Could you check a few things on this model? Use its own coordinates, in mm. Face numbers are marked on the shaded views. A direction names the side the tool comes from. Give positions to 0.01 mm unless a question says otherwise; leave off trailing zeros. Write each loop counter-clockwise with the first axis right and the second up, starting at its lowest first coordinate (ties: lowest second). Pieces come first, ordered by that corner, then holes. Notation, with made-up numbers: (37.25, 12) -> (63.25, 12) arc R22 ccw to (63.25, 28) -> close; hole circle Ø4 at (87.25, -10). An arc over 180 degrees is marked (long way). One line per question, with ' | ' between items.
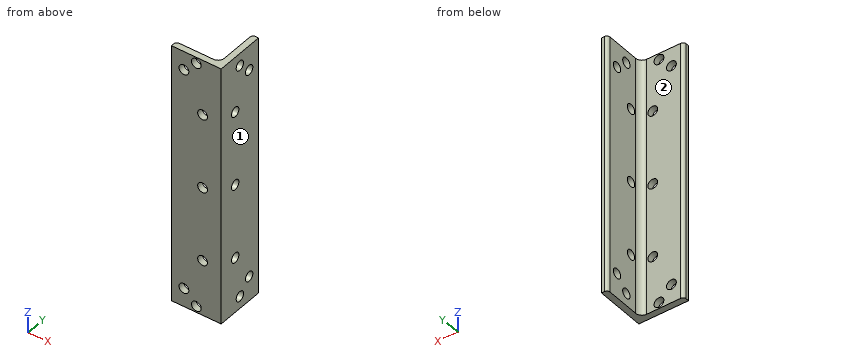
from build123d import *

# Parameters (mm, degrees)
BOSS_EXTRUDE1_DEPTH = 304.8
SKETCH7_W           = 25.4
SKETCH7_H           = 476.25
CUT_EXTRUDE1_DEPTH  = 254
SKETCH3_R           = 2.5
CUT_EXTRUDE2_DEPTH  = 254
SKETCH8_R           = 2.5
CUT_EXTRUDE4_DEPTH  = 254


with BuildPart() as part:
    # Sketch2 → Boss-Extrude1 (new, symmetric)
    with BuildSketch(Plane.XY):
        with BuildLine():
            Line((-12.7, -12.7), (12.7, -12.7))
            Line((12.7, -12.7), (12.7, 12.7))
            Line((12.7, 12.7), (11.1125, 12.7))
            ThreePointArc((11.1125, 12.7), (9.989967985, 12.235032015), (9.525, 11.1125))
            Line((9.525, 11.1125), (9.525, -6.35))
            ThreePointArc((9.525, -6.35), (8.59506403, -8.59506403), (6.35, -9.525))
            Line((6.35, -9.525), (-11.1125, -9.525))
            ThreePointArc((-11.1125, -9.525), (-12.235032015, -9.989967985), (-12.7, -11.1125))
            Line((-12.7, -11.1125), (-12.7, -12.7))
        make_face()
    extrude(amount=BOSS_EXTRUDE1_DEPTH, both=True)

    # Sketch7 → Cut-Extrude1 (cut)
    with BuildSketch(Plane.XZ.offset(12.7)):
        with Locations((0, 66.675)):
            Rectangle(SKETCH7_W, SKETCH7_H)
    extrude(amount=-CUT_EXTRUDE1_DEPTH, mode=Mode.SUBTRACT)

    # Sketch3 → Cut-Extrude2 (cut)
    with BuildSketch(Plane(origin=(0, 0, 0), x_dir=(1, 0, 0), z_dir=(0, 1, 0))):
        with Locations(Location((-6.35, 295.275, 0), (0, 0, 270))):
            Circle(SKETCH3_R)
        with Locations(Location((0, 301.625, 0), (0, 0, 270))):
            Circle(SKETCH3_R)
        with Locations(Location((3.175, 276.225, 0), (0, 0, 270))):
            Circle(SKETCH3_R)
        with Locations(Location((3.175, 238.125, 0), (0, 0, 270))):
            Circle(SKETCH3_R)
        with Locations(Location((3.175, 200.025, 0), (0, 0, 270))):
            Circle(SKETCH3_R)
        with Locations(Location((0, 174.625, 0), (0, 0, 270))):
            Circle(SKETCH3_R)
        with Locations(Location((-6.35, 180.975, 0), (0, 0, 270))):
            Circle(SKETCH3_R)
    extrude(amount=-CUT_EXTRUDE2_DEPTH, mode=Mode.SUBTRACT)

    # Sketch8 → Cut-Extrude4 (cut)
    with BuildSketch(Plane(origin=(12.7, 0, -12.7), x_dir=(0, 0, 1), z_dir=(-1, 0, 0))):
        with Locations(Location((-171.45, 6.35, 0), (0, 0, 90))):
            Circle(SKETCH8_R)
        with Locations(Location((-165.1, 0, 0), (0, 0, 90))):
            Circle(SKETCH8_R)
        with Locations(Location((-187.325, -3.175, 0), (0, 0, 90))):
            Circle(SKETCH8_R)
        with Locations(Location((-225.425, -3.175, 0), (0, 0, 90))):
            Circle(SKETCH8_R)
        with Locations(Location((-263.525, -3.175, 0), (0, 0, 90))):
            Circle(SKETCH8_R)
        with Locations(Location((-285.75, 0, 0), (0, 0, 90))):
            Circle(SKETCH8_R)
        with Locations(Location((-279.4, 6.35, 0), (0, 0, 90))):
            Circle(SKETCH8_R)
    extrude(amount=CUT_EXTRUDE4_DEPTH, mode=Mode.SUBTRACT)


solid = part.part
Q1. If I drill on line 1 along Y through (x, z) = (-8.5, -185) (3 decimals); line 2 along X through (y, z) = (4.25, -285) (3 decimals); line 3 along X through (y, z) = (-9.25, -277), over which ranges is the centre line in solid material (lowest first)?
Answer below:
line 1: y = -12.7 to -9.525 | line 2: x = 9.525 to 12.7 | line 3: x = 7.64 to 12.7
Q2. Imagine slicing it at B-B on x = -6.35. Please give me the cut outline in (y, z) (3 decimals), and give its area (3 significant figures).
Answer below:
outline: (-12.7, -304.8) -> (-9.525, -304.8) -> (-9.525, -297.775) -> (-12.7, -297.775) -> close; (-12.7, -292.775) -> (-9.525, -292.775) -> (-9.525, -183.475) -> (-12.7, -183.475) -> close; (-12.7, -178.475) -> (-9.525, -178.475) -> (-9.525, -171.45) -> (-12.7, -171.45) -> close | area: 392 mm^2
Q3. Imagine slicing it at D-D on x = 8. Please give me the cut outline in (y, z), and give its area (3 significant figures).
Answer below:
outline: (-12.7, -304.8) -> (-9.06, -304.8) -> (-9.06, -171.45) -> (-12.7, -171.45) -> close | area: 485 mm^2
Q4. Will these pins go through, and if not, where does the flat tip stop? pin 1 (8 mm diameter, centred on x = 3.175, z = -276.225, fed in from +Y); pin 2 (8 mm diameter, centred on x = -6.35, z = -180.975, fed in from +Y) (3 decimals); pin 3 (8.5 mm diameter, centred on y = 2, z = -232, fed in from -X) (3 decimals).
Answer below:
pin 1: stops at y = -9.42 | pin 2: stops at y = -9.525 | pin 3: stops at x = 9.525
Q5. Imagine slicing it at A-A on y = 6.35. Please give me the cut outline in (x, z) (3 decimals), and give its area (3 significant figures).
Answer below:
outline: (9.525, -304.8) -> (12.7, -304.8) -> (12.7, -294.6) -> (9.525, -294.6) -> close; (9.525, -289.6) -> (12.7, -289.6) -> (12.7, -186.65) -> (9.525, -186.65) -> close; (9.525, -181.65) -> (12.7, -181.65) -> (12.7, -171.45) -> (9.525, -171.45) -> close | area: 392 mm^2
Q6. On a 3-axis mill with a long thin cutter (end or side, diameter ignored), from which of +Z, -Z, +X, -X, +Y, -Y can I reach the whole of each face in a straight line? I mean the marked faces 1 and 2. Say none if no direction works.
Answer below:
face 1: +Z, -Z, +X, +Y, -Y | face 2: +Z, -Z, -X, +Y
